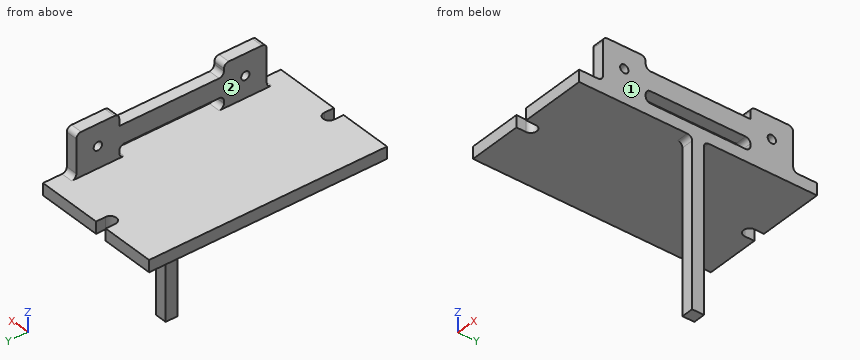
from build123d import *

# Parameters (mm, degrees)
BOSS_EXTRUDE3_DEPTH = 5
SKETCH4_W           = 5
SKETCH4_H           = 5
BOSS_EXTRUDE4_DEPTH = 70
SKETCH5_W           = 5
SKETCH5_H           = 18
BOSS_EXTRUDE5_DEPTH = 18
SKETCH6_R           = 1.75
CUT_EXTRUDE1_DEPTH  = 6
SKETCH7_W           = 8
SKETCH7_H           = 44
BOSS_EXTRUDE6_DEPTH = 5
FILLET1_R           = 2


with BuildPart() as part:
    # Sketch3 → Boss-Extrude3 (new body)
    with BuildSketch(Plane.XY):
        with BuildLine():
            Line((22.5, 100), (0, 100))
            Line((0, 100), (0, 0))
            Line((0, 0), (22.5, 0))
            Line((22.5, 0), (22.5, 4))
            ThreePointArc((22.5, 4), (25, 6.5), (27.5, 4))
            Line((27.5, 4), (27.5, 0))
            Line((27.5, 0), (55, 0))
            Line((55, 0), (55, 100))
            Line((55, 100), (27.5, 100))
            Line((27.5, 100), (27.5, 96))
            ThreePointArc((27.5, 96), (25, 93.5), (22.5, 96))
            Line((22.5, 96), (22.5, 100))
        make_face()
    extrude(amount=BOSS_EXTRUDE3_DEPTH)

    # Sketch4 → Boss-Extrude4 (add)
    with BuildSketch(Plane(origin=(0, 0, 0), x_dir=(-1, 0, 0), z_dir=(0, 0, -1))):
        with Locations((-52.5, 50)):
            Rectangle(SKETCH4_W, SKETCH4_H)
    extrude(amount=BOSS_EXTRUDE4_DEPTH)

    # Sketch5 → Boss-Extrude5 (add)
    with BuildSketch(Plane.XY.offset(5)):
        with Locations((52.5, 19)):
            Rectangle(SKETCH5_W, SKETCH5_H)
        with Locations((52.5, 81)):
            Rectangle(SKETCH5_W, SKETCH5_H)
    extrude(amount=BOSS_EXTRUDE5_DEPTH)

    # Sketch6 → Cut-Extrude1 (cut, through all)
    with BuildSketch(Plane.ZY.offset(-50)):
        with Locations((14, 19)):
            Circle(SKETCH6_R)
        with Locations((14, 81)):
            Circle(SKETCH6_R)
    extrude(amount=-CUT_EXTRUDE1_DEPTH, mode=Mode.SUBTRACT)

    # Sketch7 → Boss-Extrude6 (add)
    with BuildSketch(Plane.ZY.offset(-50)):
        with Locations((14, 50)):
            Rectangle(SKETCH7_W, SKETCH7_H)
    extrude(amount=-BOSS_EXTRUDE6_DEPTH)

    # Fillet1
    fillet1_edges = [part.edges().sort_by_distance(p)[0] for p in [
        (52.5, 47.5, 0),
        (52.5, 52.5, 0),
        (52.5, 10, 5),
        (52.5, 28, 5),
        (52.5, 10, 23),
        (52.5, 28, 23),
        (52.5, 72, 5),
        (52.5, 90, 5),
        (52.5, 72, 23),
        (52.5, 90, 23),
        (52.5, 72, 10),
        (52.5, 28, 10),
        (52.5, 28, 18),
    ]]
    fillet(fillet1_edges, radius=FILLET1_R)


solid = part.part
Model file for the job. Use its own axes, mm. Face numbers are marked on the shaded views. A direction names the side the tool comes from. Give positions to 0.01 mm unless a question says otherwise; leave off trailing zeros. Loops run counter-clockwise (first coordinate to the right, second up) from the corner with the lowest first, then second, coordinate; pieces in that order, holes last.
Item 1: Slice it at C-C (y = 33.5). Write the cut outline in (x, z).
Check values:
outline: (0, 0) - (55, 0) - (55, 5) - (0, 5) - close; (50, 10) - (55, 10) - (55, 18) - (50, 18) - close
Item 2: Slice it at D-D (z = -53). Write the cut outline in (x, y), plus the area to 3 significant figures.
Check values:
outline: (50, 47.5) - (55, 47.5) - (55, 52.5) - (50, 52.5) - close
area: 25.0 mm2
Item 3: Which spindle directions (+Z, -Z, +X, -X, +Y, -Y) get a long thin tool onto all of the face, cutting with end or side? Do the marked faces 1 and 2. Say none if no direction does.
Check values:
face 1: +Z, -Z, +X, +Y, -Y
face 2: +Z, -X, +Y, -Y
Item 4: Slice it at B-B (x = 25). Write the cut outline in (y, z).
Check values:
outline: (6.5, 0) - (93.5, 0) - (93.5, 5) - (6.5, 5) - close
Item 5: Drop flat-ended pins along their axis: P1, Ø6, axis at x = 40.5, y = 40, coming from the +Z side; P2, Ø2.5, axis at x = 52.5, z = 19, coming from the -Y side; P3, Ø5.5, axis at y = 19, z = 14, coming from the -X side. Give the stop position or say it passes through.
Check values:
P1: stops at z = 5
P2: stops at y = 10
P3: stops at x = 50
Item 6: Slice it at A-A (y = 81). Write the cut outline in (x, z), plus the area to 4 significant figures.
Check values:
outline: (0, 0) - (55, 0) - (55, 12.25) - (50, 12.25) - (50, 5) - (0, 5) - close; (50, 15.75) - (55, 15.75) - (55, 23) - (50, 23) - close
area: 347.5 mm2
Item 7: Drill centre lines: line 1 along Y through (x, z) = (51, 14); line 2 along Z through (x, y) = (51.15, 81); line 3 along Z through (x, y) = (47.5, 64.5). Where is each one in solid material? Low to high.
Check values:
line 1: y = 10 to 17.25, 20.75 to 79.25, 82.75 to 90
line 2: z = 0 to 12.25, 15.75 to 23
line 3: z = 0 to 5
